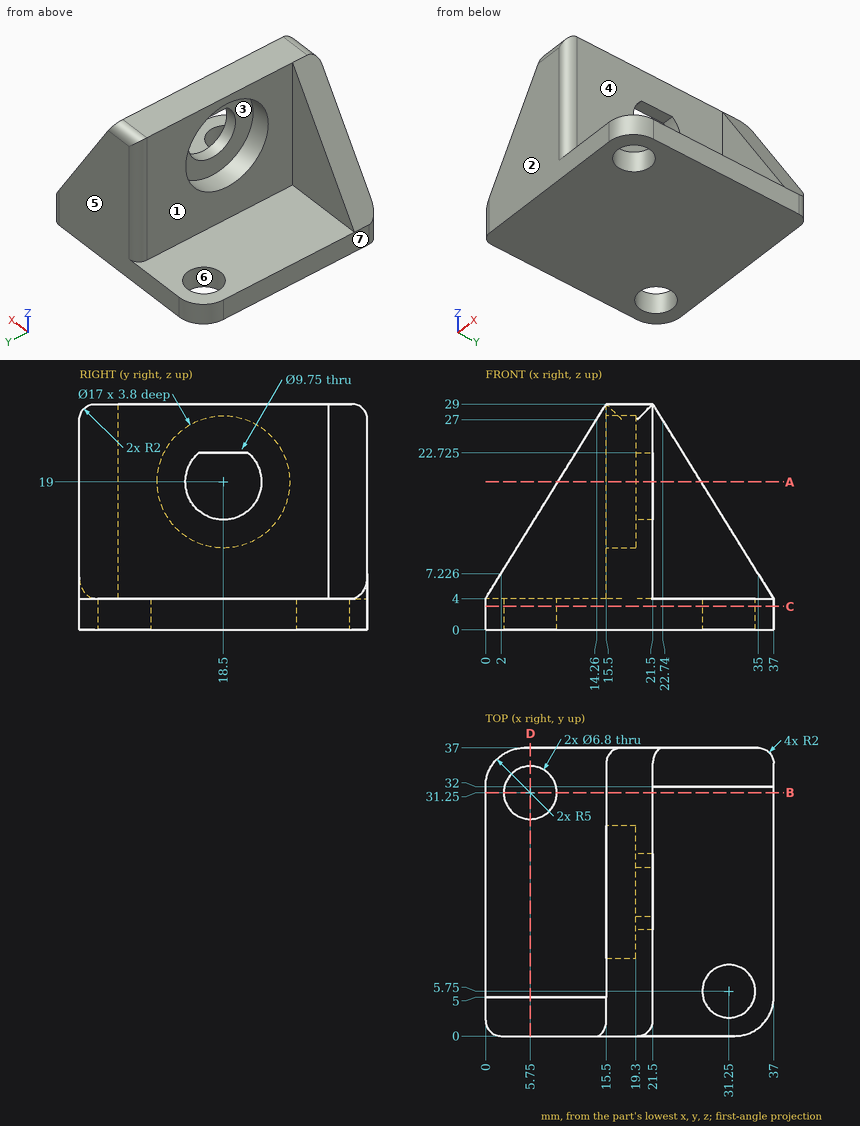
Print and shaded views of the part. All mm, measured from the part's lowest x, y and z. A direction names the side the tool comes from. Round coordinates to 2 decimals unless told otherwise and drop trailing zeros. Loops run counter-clockwise (first coordinate to the right, second up) from the corner with the lowest first, then second, coordinate; pieces in that order, holes last. Notation, with made-up numbers: (-31, -5) -> (-9, -5) arc R29 cw to (-9, 15) -> close; hole circle Ø2 at (23, 86). An arc over 180 degrees is marked (long way). Use CSV: the item, a comma, the result in double quotes. Start each with the question number.
1) Cut at B-B, the plane y = 31.25. Write the cut outline in (x, z), plus the area to 3 significant figures.
2) Wall check: L1, parallel to Z at x = 17.5, y = 18.5; L2, parallel to X at y = 11, z = 26.75; L3, parallel to Y at x = 12.5, z = 13.5. Give the ranges that are in metal, low to high. Write a range as [from, to].
3) Pull direction Y, two halves, no side cores. Call the marked faces 5, 6 and 7: +Y half, -Y half, draft (parallel to the pull), parting line (faces both ways), or undercut.
4) Drop flat-ended pins along their axis: P1, Ø1.1, axis at x = 20, y = 19.5, coming from the -Z side; P2, Ø6, axis at x = 31.25, y = 5.75, coming from the -Z side; P3, Ø11, axis at y = 18.5, z = 19, coming from the +X side; P4, Ø4.5, axis at x = 6, z = 14, coming from the +Y side. Give the stop position or say it passes through.
5) Cut at A-A, the plane z = 19. Write the cut outline in (x, y) (3 decimals).
6) Cut at D-D, the plane x = 5.75. Write the cut outline in (y, z), plus the area to 3 significant figures.
7) Which spindle directions (+Z, -Z, +X, -X, +Y, -Y) get a long thin tool onto all of the face, cutting with end or side? Do the marked faces 1, 2, 3 and 4. Say none if no direction does.
8) Cut at C-C, the plane z = 3. Write the cut outline in (x, y).
Determined:
1,outline,"(0, 0) -> (2.35, 0) -> (2.35, 4) -> (0, 4) -> close; (9.15, 0) -> (37, 0) -> (37, 4) -> (21.5, 4) -> (21.5, 29) -> (15.5, 29) -> (15.5, 4) -> (9.15, 4) -> close"
1,area,"271 mm2"
2,L1,"z = [0, 10.5], [27.5, 29]"
2,L2,"x = [15.5, 21.5]"
2,L3,"y = [0, 5]"
3,face 5,"+Y half"
3,face 6,"undercut"
3,face 7,"draft"
4,P1,"stops at z = 0"
4,P2,"passes through"
4,P3,"stops at x = 21.5"
4,P4,"stops at y = 5"
5,outline,"(9.3, 0) -> (19.5, 0) arc R2 ccw to (21.5, 2) -> (21.5, 13.625) -> (19.3, 13.625) -> (19.3, 10) -> (15.5, 10) -> (15.5, 5) -> (9.3, 5) -> close; (15.5, 27) -> (19.3, 27) -> (19.3, 23.375) -> (21.5, 23.375) -> (21.5, 32) -> (27.7, 32) -> (27.7, 37) -> (17.5, 37) arc R2 ccw to (15.5, 35) -> close"
6,outline,"(0, 0) -> (27.85, 0) -> (27.85, 4) -> (5, 4) -> (5, 13.27) -> (0, 13.27) -> close; (34.65, 0) -> (37, 0) -> (37, 4) -> (34.65, 4) -> close"
6,area,"167 mm2"
7,face 1,"+Z, -X, +Y"
7,face 2,"+Z, -Z, +X, -X, -Y"
7,face 3,"-X"
7,face 4,"+Z, +X, -Y"
8,outline,"(0, 2) arc R2 ccw to (2, 0) -> (32, 0) arc R5 ccw to (37, 5) -> (37, 35) arc R2 ccw to (35, 37) -> (5, 37) arc R5 ccw to (0, 32) -> close; hole circle Ø6.8 at (5.75, 31.25); hole circle Ø6.8 at (31.25, 5.75)"
